from build123d import *

# Parameters (mm, degrees)
EXTRUDE_1_DEPTH     = 3
CUT_EXTRUDE_1_DEPTH = 0.8
CUT_EXTRUDE_2_DEPTH = 4.7


with BuildPart() as part:
    # Эскиз1 → Бобышка-Вытянуть1 (new body, symmetric)
    with BuildSketch(Plane.XY):
        Polygon((3, 0), (-3, 0), (-3, -0.8), (-5, -0.8), (-5, -4.5), (5, -4.5), (5, -0.8), (3, -0.8), align=None)
    extrude(amount=EXTRUDE_1_DEPTH, both=True)

    # Эскиз3 → Отверстие обработанное метчиком M51 (revolve, cut)
    with BuildSketch(Plane(origin=(0, 0, 0), x_dir=(0, 0, 1), z_dir=(1, 0, 0))):
        Polygon((0, 0), (0, 4.5), (2.6, 4.5), (2.1, 4), (2.1, 0.5), (2.6, 0), align=None)
    revolve(axis=Axis((0, 6.35, 0), (0, -1, 0)), mode=Mode.SUBTRACT)

    # Эскиз4 → Вырез-Вытянуть1 (cut)
    with BuildSketch(Plane(origin=(0, 0, 0), x_dir=(1, 0, 0), z_dir=(0, 1, 0))):
        with BuildLine():
            Line((-3, 3), (-3, 0))
            ThreePointArc((-3, 0), (-2.121320344, 2.121320344), (0, 3))
            Line((0, 3), (-3, 3))
        make_face()
        with BuildLine():
            Line((0, -3), (3, -3))
            Line((3, -3), (3, 0))
            ThreePointArc((3, 0), (2.121320344, -2.121320344), (0, -3))
        make_face()
    extrude(amount=-CUT_EXTRUDE_1_DEPTH, mode=Mode.SUBTRACT)

    # Эскиз5 → Вырез-Вытянуть2 (cut, through all)
    with BuildSketch(Plane(origin=(0, -0.8, 0), x_dir=(1, 0, 0), z_dir=(0, 1, 0))):
        with BuildLine():
            Line((-5, 0), (-5, 3))
            Line((-5, 3), (-4, 3))
            ThreePointArc((-4, 3), (-4.74341649, 1.58113883), (-5, 0))
        make_face()
        with BuildLine():
            Line((5, 0), (5, -3))
            Line((5, -3), (4, -3))
            ThreePointArc((4, -3), (4.74341649, -1.58113883), (5, 0))
        make_face()
    extrude(amount=-CUT_EXTRUDE_2_DEPTH, mode=Mode.SUBTRACT)

    # Вырез-По траектории1: sweep along a path in Эскиз7
    with BuildLine(Plane.XZ.offset(4.5)) as sweep_1_path:
        Line((0, 5), (-5, 5))
        Line((-5, 5), (-5, 0))
        ThreePointArc((-5, 0), (-3.535533906, -3.535533906), (0, -5))
        Line((0, -5), (5, -5))
        Line((5, -5), (5, 0))
        ThreePointArc((5, 0), (3.535533906, 3.535533906), (0, 5))
    # Эскиз6 → Вырез-По траектории1 (sweep, cut)
    with BuildSketch(Plane.XY.offset(3)):
        Polygon((-5, -2.3), (-5, -4.5), (-3, -4.5), align=None)
    sweep(path=sweep_1_path.line, transition=Transition.RIGHT, mode=Mode.SUBTRACT)


solid = part.part
Check sheet for the modelled part. Datum: model origin and axes. Units: mm. A direction names the side the tool comes from. Give positions to 0.01 mm unless a question says otherwise; leave off trailing zeros. Order: outer loops, then holes, each group sorted by start corner. A loop starts at its lowest first (then second) coordinate and runs counter-clockwise, first axis right, second up. Notation, with made-up numbers: M 30,60.25 L 67,60.25 A13 ccw 67,73.25 Z; hole C 84.5,62.5 d5. An arc over 180 degrees is marked long. Answer as CSV lines item,"result". Start each with the question number.
Item 1: Gauge pin test, flat end, axial feed: P1, Ø1, axis at y = -2.5, z = 1, coming from the +X side. Record the tip position at first contact, or that the pin passes through.
Item 2: Cross-section at A-A on y = -1.15. Enter the section's corners in (x, z), plus the area to 3 significant figures.
Item 3: Tool access check on faces 1 (the face through (-2.14, -0.39, -2.1)), 2 (the face through (0, -2, -3)). Record the directions out of +Z, -Z, +X, -X, +Y, -Y that give a thin tool (end or side, any length) a straight path to the whole face; none if there is none.
Item 4: Mould release check, pull along X, two halves, no side actions. Record for faces 3 (the face through (-4, -0.8, 0)), 4 (the face through (-3.454, -3.629, -1.565)), 5 (the face through (2.14, -0.39, 2.1)), 6 (the face through (-0.631, -2.226, 2.003)): +X half, -X half, draft (parallel to the pull), parting line (faces both ways), or undercut.
Item 5: Cross-section at B-B on y = -3.4. Enter the section's corners in (x, z), plus the area to 3 significant figures.
Item 6: Thickness scan on line 1 (Z direction, x = 0, y = -1.75); line 2 (Z direction, x = 1.5, y = -3.4); line 3 (X direction, y = -3.1, z = 0). Record the ranges inside material, lowest first. Write a range as [from, to].
Established:
1,P1,"stops at x = 4.97"
2,outline,"M -5,0 A5 ccw -4,-3 L 5,-3 L 5,0 A5 ccw 4,3 L -5,3 Z; hole C 0,0 d4.2"
2,area,"44.2 mm^2"
3,face 1,"-Z, -X, +Y"
3,face 2,"-Z, +X, -X, +Y, -Y"
4,face 3,"draft"
4,face 4,"-X half"
4,face 5,"+X half"
4,face 6,"undercut"
5,outline,"M -4,0 A4 ccw -2.65,-3 L 4,-3 L 4,0 A4 ccw 2.65,3 L -4,3 Z; hole C 0,0 d4.2"
5,area,"31.7 mm^2"
6,line 1,"z = [-3, -2.1], [2.1, 3]"
6,line 2,"z = [-3, -1.47], [1.47, 3]"
6,line 3,"x = [-4.27, -2.1], [2.1, 4.27]"
